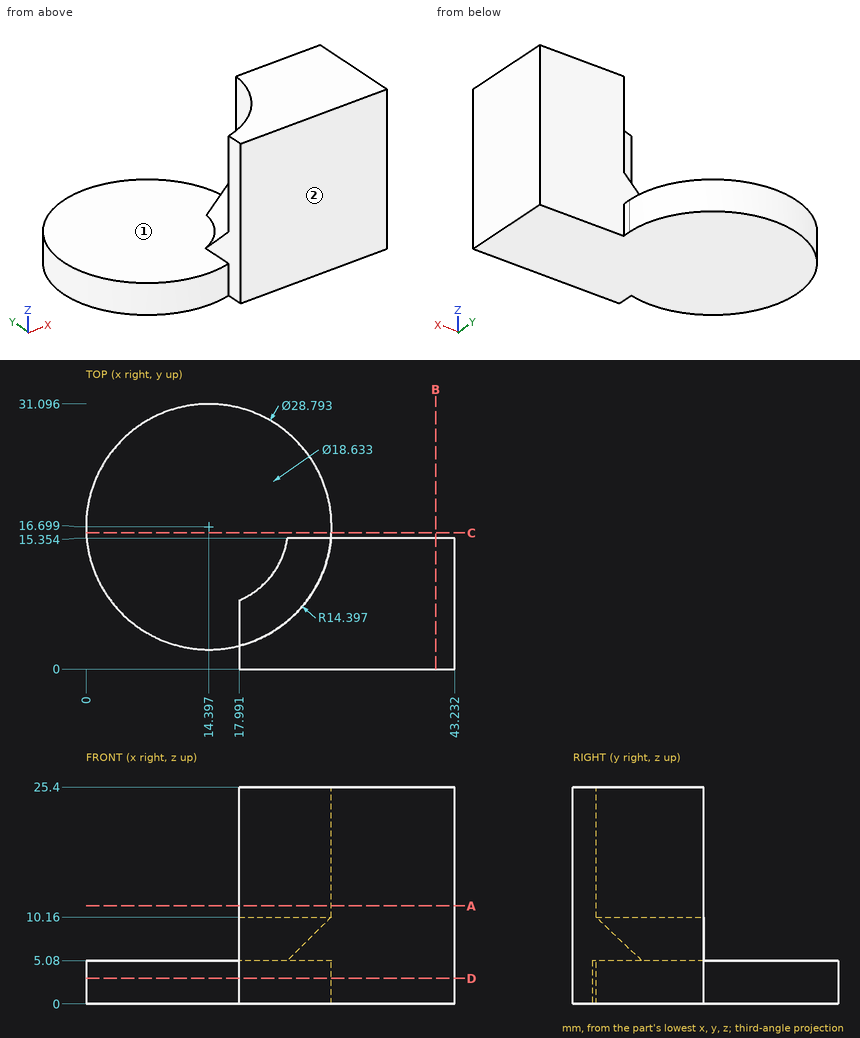
Input: dimensioned drawing with shaded views. Units: mm. Origin: part minimum x, y, z. A direction names the side the tool comes from. Coordinates: 2 decimals unless noted, no trailing zeros. Loops run counter-clockwise (first coordinate to the right, second up) from the corner with the lowest first, then second, coordinate; pieces in that order, holes last. Notation, with made-up numbers: (86, 83.25) -> (93, 83.25) arc R10 cw to (93, 101.25) -> close; hole circle Ø2 at (86, -19). An arc over 180 degrees is marked (long way). Use a Markdown table: item, result. Add a question column.
(1) Line query: line 1 along Z through (x, y) = (11, 8.5); line 2 along Y through (x, z) = (34, 5.25); line 3 along X through (y, z) = (2, 15.75). Output: solid intervals per line, ascending.
(2) Pin query (flat end, axial travel): pin 1 Ø5 at (x, z) = (30, 19.5) entering from +Y; pin 2 Ø8 at (y, z) = (27.5, 10) entering from -X; pin 3 Ø4 at (y, z) = (4, 17) entering from -X. Return the tip coordinate at first contact, or that it passes through.
(3) Section query A-A, the plane z = 11.5. Return loops of the section in (x, y).
(4) Section query C-C, the plane y = 16. Return loops of the section in (x, z), plus the area to 3 significant figures.
(5) Access query for the marked faces 1 and 2. Directions: +Z, -Z, +X, -X, +Y, -Y. A direction counts if a zero-diameter tool reaches every point of the face in a straight line with its end or side. Return the directions, or none.
(6) Section query B-B, the plane x = 41. Return loops of the section in (y, z).
(7) Section query D-D, the plane z = 3. Return loops of the section in (x, y).
Answer:
| question | item | result |
|---|---|---|
| 1 | line 1 | z = 0 to 5.08 |
| 1 | line 2 | y = 0 to 15.35 |
| 1 | line 3 | x = 17.99 to 43.23 |
| 2 | pin 1 | stops at y = 15.35 |
| 2 | pin 2 | passes through |
| 2 | pin 3 | stops at x = 17.99 |
| 3 | outline | (17.99, 0) -> (43.23, 0) -> (43.23, 15.35) -> (28.73, 15.35) arc R14.4 cw to (17.99, 2.76) -> close |
| 4 | outline | (0.02, 0) -> (28.78, 0) -> (28.78, 5.08) -> (0.02, 5.08) -> close |
| 4 | area | 146 mm^2 |
| 5 | face 1 | +Z, -X, +Y |
| 5 | face 2 | +Z, -Z, +X, -X, -Y |
| 6 | outline | (0, 0) -> (15.35, 0) -> (15.35, 25.4) -> (0, 25.4) -> close |
| 7 | outline | (17.99, 0) -> (43.23, 0) -> (43.23, 15.35) -> (28.73, 15.35) arc R14.4 ccw (long way) to (17.99, 2.76) -> close |
